```python
from build123d import *

# Parameters (mm, degrees)
F1_DEPTH    = 10
F2_T1_DEPTH = 29
F2_T3_DEPTH = 29
F3_R        = 5
F4_DEPTH    = 25.4


# Not quite as in the source:
# - a fillet or chamfer that OpenCascade refuses, or shapes differently, is made with other operations: its cross-section is extruded or revolved along the edge and cut away or added


with BuildPart() as f1:
    # F0 (on Front) → F1 (new body, symmetric)
    with BuildSketch(Plane.XZ):
        with BuildLine():
            Line((-70, -10), (-48.9897948557, -10))
            ThreePointArc((-48.9897948557, -10), (50, 0), (-48.9897948557, 10))
            Line((-48.9897948557, 10), (-70, 10))
            Line((-70, 10), (-70, 6))
            Line((-70, 6), (-45.607017004, 6))
            ThreePointArc((-45.607017004, 6), (46, 0), (-45.607017004, -6))
            Line((-45.607017004, -6), (-70, -6))
            Line((-70, -6), (-70, -10))
        make_face()
    extrude(amount=F1_DEPTH, both=True)

    # F2: fillet of radius 5 on 4 edges, made by hand

    # F2_s2 → F2_t1 (cut)
    with BuildSketch(Plane.XY.offset(-6.5)):
        with BuildLine():
            add(Edge.make_bspline(
                [(-70, 5), (-70, 10), (-65, 10)],
                knots=[0, 0, 0, 1, 1, 1], degree=2, weights=[1, 1, 1]))
            Line((-65, 10), (-70, 10))
            Line((-70, 10), (-70, 5))
        make_face()
        with BuildLine():
            add(Edge.make_bspline(
                [(-70, -5), (-70, -10), (-65, -10)],
                knots=[0, 0, 0, 1, 1, 1], degree=2, weights=[1, 1, 1]))
            Line((-65, -10), (-70, -10))
            Line((-70, -10), (-70, -5))
        make_face()
    extrude(amount=F2_T1_DEPTH, mode=Mode.SUBTRACT)

    # F2_s4 → F2_t3 (cut)
    with BuildSketch(Plane.XY.offset(-22.5)):
        with BuildLine():
            add(Edge.make_bspline(
                [(-70, 5), (-70, 10), (-65, 10)],
                knots=[0, 0, 0, 1, 1, 1], degree=2, weights=[1, 1, 1]))
            Line((-65, 10), (-70, 10))
            Line((-70, 10), (-70, 5))
        make_face()
        with BuildLine():
            add(Edge.make_bspline(
                [(-65, -10), (-70, -10), (-70, -5)],
                knots=[0, 0, 0, 1, 1, 1], degree=2, weights=[1, 1, 1]))
            Line((-70, -5), (-70, -10))
            Line((-70, -10), (-65, -10))
        make_face()
    extrude(amount=F2_T3_DEPTH, mode=Mode.SUBTRACT)

    # F3 (on face) → F4 (cut)
    with BuildSketch(Plane.XY.offset(10)):
        with Locations((-60, 0)):
            Circle(F3_R)
    extrude(amount=-F4_DEPTH, mode=Mode.SUBTRACT)


solid = f1.part
```
For this review, take the finished solid that the model builds, in its own axes (mm). A direction names the side the tool comes from. Coordinates: 2 decimals unless noted, no trailing zeros. Write each loop counter-clockwise with the first axis right and the second up, starting at its lowest first coordinate (ties: lowest second). Pieces come first, ordered by that corner, then holes. Notation, with made-up numbers: (79, -24.75) - (97, -24.75) arc R26 ccw to (97, -8.75) - close; hole circle Ø4 at (60.25, -9.75). An arc over 180 degrees is marked (long way). Answer in a Markdown table with one row per item. Add a question column.
Q1. Tool access review of faces 1 (the flat face through (-70, 0, 8)), 2 (the cylindrical face through (49.958, -0.14, -2.058)), 3 (the flat face through (-55, 2, -10)), 4 (the flat face through (-55, 2, -6)), 5 (the flat face through (-54.7, -0.1, 10)): name each direction out of +Z, -Z, +X, -X, +Y, -Y from which nothing blocks a thin tool from reaching the whole face with its end or side.
Q2. Draft analysis for pull direction Y (two halves, no side actions). For faces 6 (the cylindrical face through (-65, 0, 8)), 7 (the flat face through (-70, 0, -8)), 8 (the flat face through (-46, -10, -7)), state which applies: +Y half, -Y half, draft (parallel to the pull), parting line (faces both ways), or undercut.
Q3. We need section A-A, the plane x = -60. State the section outline as (y, z) points, and give its area (3 significant figures).
Q4. We need section D-D, the plane x = 32.5. State the section outline as (y, z) points.
Q5. For P1, Ø12, axis at x = 15.5, y = 4, coming from the -Z side; P2, Ø6, axis at x = -6, y = -5, coming from the +Z side; P3, Ø10, axis at x = -63.5, y = -3, coming from the -Z side, all flat-tipped, find the tip position at first contact; note any pin that passes through.
Q6. We need section B-B, the plane y = -3. State the section outline as (x, z) points.
Q7. We need section C-C, the plane z = 31. State the section outline as (x, y) points, and give its area (3 significant figures).
Q8. For probe 1 along Y at (x, z) = (-60, -9); probe 2 along X at (y, z) = (-4, -8.5); probe 3 along X at (y, z) = (0.25, 35.5), list the stretches that pass through material, from the lowest coordinate up.
Answer list:
| question | item | result |
|---|---|---|
| 1 | face 1 | +Z, -Z, -X, +Y, -Y |
| 1 | face 2 | +Y, -Y |
| 1 | face 3 | -Z, -X, +Y, -Y |
| 1 | face 4 | -X, +Y, -Y |
| 1 | face 5 | +Z, -X, +Y, -Y |
| 2 | face 6 | undercut |
| 2 | face 7 | draft |
| 2 | face 8 | -Y half |
| 3 | outline | (-10, -10) - (-5, -10) - (-5, -6) - (-10, -6) - close; (-10, 6) - (-5, 6) - (-5, 10) - (-10, 10) - close; (5, -10) - (10, -10) - (10, -6) - (5, -6) - close; (5, 6) - (10, 6) - (10, 10) - (5, 10) - close |
| 3 | area | 80.0 mm2 |
| 4 | outline | (-10, -38) - (10, -38) - (10, -32.55) - (-10, -32.55) - close; (-10, 32.55) - (10, 32.55) - (10, 38) - (-10, 38) - close |
| 5 | P1 | stops at z = -49.09 |
| 5 | P2 | stops at z = 49.91 |
| 5 | P3 | stops at z = -10 |
| 6 | outline | (-70, -10) - (-64, -10) - (-64, -6) - (-70, -6) - close; (-70, 6) - (-64, 6) - (-64, 10) - (-70, 10) - close; (-56, -10) - (-48.99, -10) arc R50 ccw (long way) to (-48.99, 10) - (-56, 10) - (-56, 6) - (-45.61, 6) arc R46 cw (long way) to (-45.61, -6) - (-56, -6) - close |
| 7 | outline | (-39.23, -10) - (-33.99, -10) - (-33.99, 10) - (-39.23, 10) - close; (33.99, -10) - (39.23, -10) - (39.23, 10) - (33.99, 10) - close |
| 7 | area | 210 mm2 |
| 8 | probe 1 | y = -10 to -5, 5 to 10 |
| 8 | probe 2 | x = -70 to -63, -57 to -45.21, 45.21 to 49.27 |
| 8 | probe 3 | x = -35.21 to -29.25, 29.25 to 35.21 |
